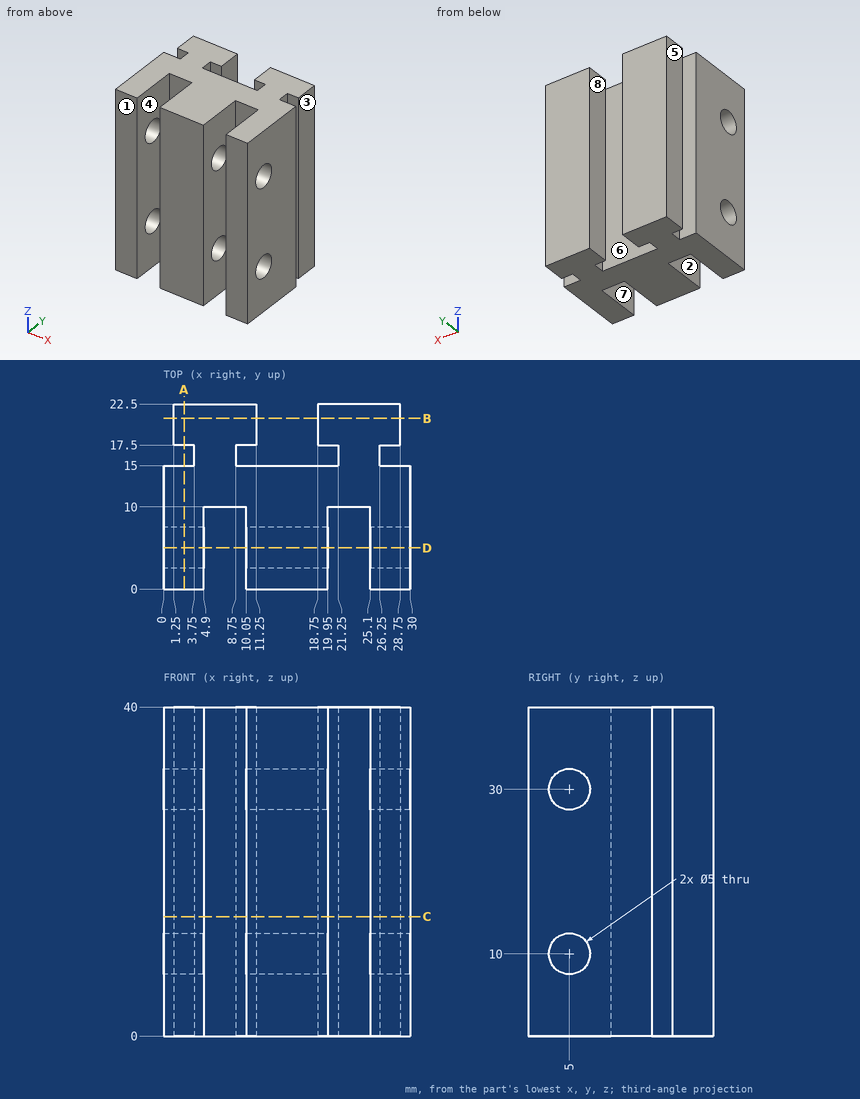
Verification items for this drawing (mm, ordinates from the low corner). A direction names the side the tool comes from. Give positions to 0.01 mm unless a question says otherwise; leave off trailing zeros. Order: outer loops, then holes, each group sorted by start corner. A loop starts at its lowest first (then second) coordinate and runs counter-clockwise, first axis right, second up. Notation, with made-up numbers: M 86,2 L 95,2 A15 cw 95,15 Z; hole C 30,-36 d10. An arc over 180 degrees is marked long. Use a Markdown table: item, result.
Item 1: Material ranges on line 1 along Y through (x, z) = (26.35, 10); line 2 along X through (y, z) = (9.75, 20.5); line 3 along Y through (x, z) = (14.5, 30), recorded low to high.
Answers follow:
| item | result |
|---|---|
| line 1 | y = 0 to 2.5, 7.5 to 15, 17.5 to 22.5 |
| line 2 | x = 0 to 4.9, 10.05 to 19.95, 25.1 to 30 |
| line 3 | y = 0 to 2.5, 7.5 to 15 |
Item 2: Section check C-C (z = 14.5). Record the cut outline in (x, y), and give its area (3 significant figures).
Answers follow:
| item | result |
|---|---|
| outline | M 0,0 L 4.9,0 L 4.9,10 L 10.05,10 L 10.05,0 L 19.95,0 L 19.95,10 L 25.1,10 L 25.1,0 L 30,0 L 30,15 L 26.25,15 L 26.25,17.5 L 28.75,17.5 L 28.75,22.5 L 18.75,22.5 L 18.75,17.5 L 21.25,17.5 L 21.25,15 L 8.75,15 L 8.75,17.5 L 11.25,17.5 L 11.25,22.5 L 1.25,22.5 L 1.25,17.5 L 3.75,17.5 L 3.75,15 L 0,15 Z |
| area | 472 mm2 |
Item 3: Section check B-B (y = 20.75). Record the cut outline in (x, z).
Answers follow:
| item | result |
|---|---|
| outline | M 1.25,0 L 11.25,0 L 11.25,40 L 1.25,40 Z; M 18.75,0 L 28.75,0 L 28.75,40 L 18.75,40 Z |
Item 4: Depth check by flat-ended pin: P1, Ø1.5, axis at x = 7, z = 10.5, coming from the -Y side; P2, Ø4, axis at y = 20, z = 12.5, coming from the -X side; P3, Ø4, axis at y = 19, z = 10.5, coming from the +X side. Enter the tip coordinate at first touch or a pass-through.
Answers follow:
| item | result |
|---|---|
| P1 | stops at y = 10 |
| P2 | stops at x = 1.25 |
| P3 | stops at x = 28.75 |
Item 5: Draft check along X on the marked faces 1, 2, 3 and 4. Enter one of: +X half, -X half, draft (parallel to the pull), parting line (faces both ways), or undercut.
Answers follow:
| item | result |
|---|---|
| face 1 | draft |
| face 2 | undercut |
| face 3 | +X half |
| face 4 | undercut |
Item 6: Section check A-A (x = 2.5). Record the cut outline in (y, z).
Answers follow:
| item | result |
|---|---|
| outline | M 0,0 L 15,0 L 15,40 L 0,40 Z; M 17.5,0 L 22.5,0 L 22.5,40 L 17.5,40 Z; hole C 5,10 d5; hole C 5,30 d5 |
Item 7: Tool access check on the marked faces 5, 6, 7 and 8. Record the directions out of +Z, -Z, +X, -X, +Y, -Y that give a thin tool (end or side, any length) a straight path to the whole face; none if there is none.
Answers follow:
| item | result |
|---|---|
| face 5 | +Z, -Z, -X, +Y |
| face 6 | +Z, -Z |
| face 7 | +Z, -Z, -Y |
| face 8 | +Z, -Z, +Y |
Item 8: Section check D-D (y = 5). State how many separate pieces and enclosed holes the cut face has, and give its area (3 significant figures).
Answers follow:
| item | result |
|---|---|
| separate pieces | 9 |
| enclosed holes | 0 |
| area | 591 mm2 |
